Input: dimensioned drawing with shaded views. Units: mm. Origin: part minimum x, y, z. A direction names the side the tool comes from. Round coordinates to 2 decimals unless told otherwise and drop trailing zeros. Write each loop counter-clockwise with the first axis right and the second up, starting at its lowest first coordinate (ties: lowest second). Pieces come first, ordered by that corner, then holes. Notation, with made-up numbers: (85.25, 34) -> (91.25, 34) arc R37 ccw to (91.25, 71) -> close; hole circle Ø7 at (3, -11). An arc over 180 degrees is marked (long way). Return JSON: item names as keys, results as strings. Group by question number.
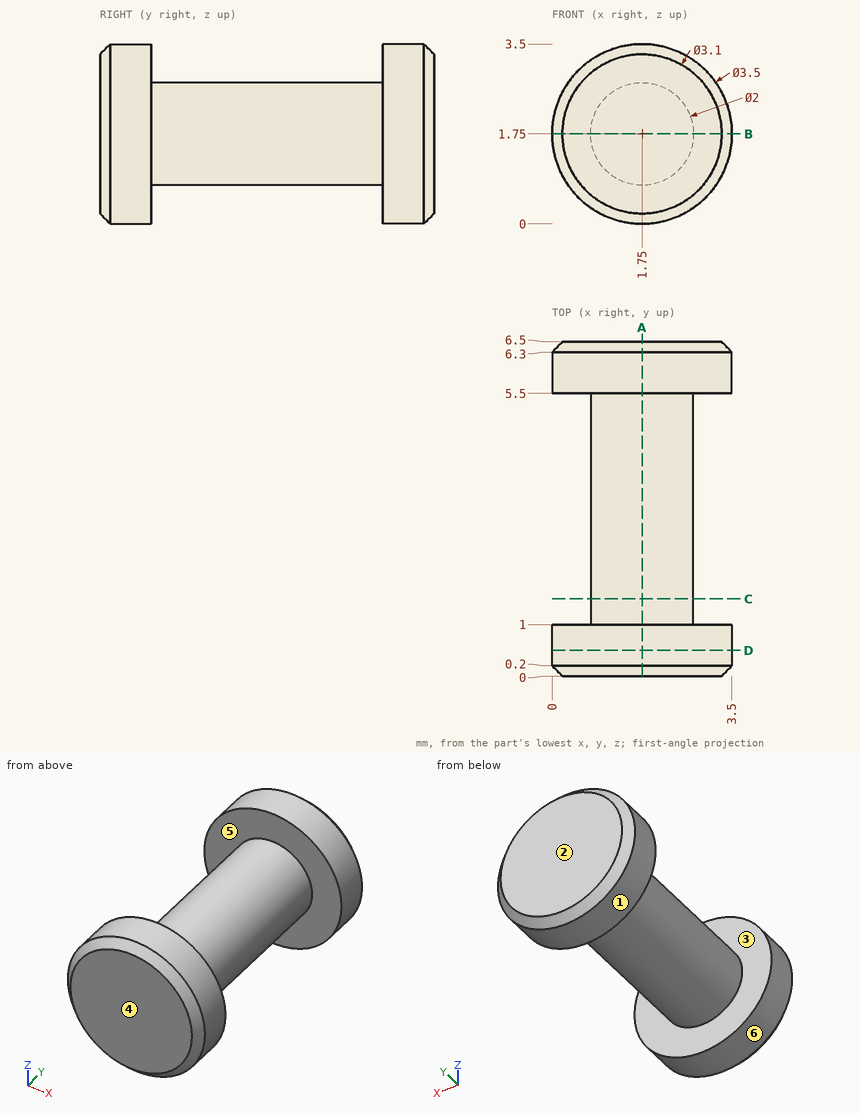
Item 1: First-contact query: pin 1 Ø1 at (y, z) = (4.5, 2.5) entering from +X; pin 2 Ø1.5 at (y, z) = (3, 1.5) entering from -X. Flat tips, straight axial feed; report the tip coordinate or a pass-through.
Item 2: Set-up query: the marked faces 5 and 6. Return all of +Z, -Z, +X, -X, +Y, -Y with unobstructed straight access to the full face (end or side cutting, diameter ignored); none if empty.
Item 3: Cut plane D-D on y = 0.5. Output: boundary loops of the cut face in (x, z), and give its area (3 significant figures).
Item 4: Cut plane C-C on y = 1.5. Output: boundary loops of the cut face in (x, z), and give its area (3 significant figures).
Item 5: Cut plane A-A on x = 1.75. Output: boundary loops of the cut face in (y, z), and give its area (3 significant figures).
Item 6: Material intervals for probe 1 along Y at (x, z) = (0.65, 2.1); probe 2 along X at (y, z) = (4.5, 1.4); probe 3 along X at (y, z) = (0.5, 1.9), sorted ascending.
Item 7: Cut plane B-B on z = 1.75. Output: boundary loops of the cut face in (x, y).
Item 8: Pull-direction query (Y, two-part tool) for the marked faces 1, 2, 3 and 4; classes: +Y half, -Y half, draft (parallel to the pull), parting line (faces both ways), or undercut.
Here are the results:
{
 "1": {"pin 1": "stops at x = 2.72", "pin 2": "stops at x = 0.75"},
 "2": {"face 5": "none", "face 6": "+Y, -Y"},
 "3": {"outline": "circle Ø3.5 at (1.75, 1.75)", "area": "9.62 mm^2"},
 "4": {"outline": "circle Ø2 at (1.75, 1.75)", "area": "3.14 mm^2"},
 "5": {"outline": "(0, 0.2) -> (0.2, 0) -> (1, 0) -> (1, 0.75) -> (5.5, 0.75) -> (5.5, 0) -> (6.3, 0) -> (6.5, 0.2) -> (6.5, 3.3) -> (6.3, 3.5) -> (5.5, 3.5) -> (5.5, 2.75) -> (1, 2.75) -> (1, 3.5) -> (0.2, 3.5) -> (0, 3.3) -> close", "area": "15.9 mm^2"},
 "6": {"probe 1": "y = 0 to 1, 5.5 to 6.5", "probe 2": "x = 0.81 to 2.69", "probe 3": "x = 0.01 to 3.49"},
 "7": {"outline": "(0, 0.2) -> (0.2, 0) -> (3.3, 0) -> (3.5, 0.2) -> (3.5, 1) -> (2.75, 1) -> (2.75, 5.5) -> (3.5, 5.5) -> (3.5, 6.3) -> (3.3, 6.5) -> (0.2, 6.5) -> (0, 6.3) -> (0, 5.5) -> (0.75, 5.5) -> (0.75, 1) -> (0, 1) -> close"},
 "8": {"face 1": "draft", "face 2": "+Y half", "face 3": "undercut", "face 4": "-Y half"}
}
